Geometry check sheet. Reference: the model listing, model coordinates, mm. Round coordinates to 2 decimals unless told otherwise and drop trailing zeros. Loops run counter-clockwise (first coordinate to the right, second up) from the corner with the lowest first, then second, coordinate; pieces in that order, holes last. Notation, with made-up numbers: (-8, 78) -> (-4, 78) arc R23 cw to (-4, 99) -> close; hole circle Ø7 at (40.5, 3). An arc over 180 degrees is marked (long way). Use one line per item in the form item = value.
from build123d import *

# Parameters (mm, degrees)
EXTRUDE_2_DEPTH     = 2.5
SKETCH_2_R          = 1.5
CUT_EXTRUDE_1_DEPTH = 81.816149376


with BuildPart() as part:
    # 草图1 → 凸台-拉伸2 (new body)
    with BuildSketch(Plane(origin=(0, 0, 0), x_dir=(1, 0, 0), z_dir=(0, 1, 0))):
        Polygon((0, -30), (0, 30), (75, 30), (75, 10), (65, 10), (65, 20), (10, 20), (10, -20), (65, -20), (65, -10), (75, -10), (75, -30), align=None)
    extrude(amount=EXTRUDE_2_DEPTH)

    # 草图2 → 切除-拉伸1 (cut, through all)
    with BuildSketch(Plane(origin=(0, 0, 0), x_dir=(1, 0, 0), z_dir=(0, 1, 0))):
        with Locations(Location((5, 25, 0), (0, 0, 270))):
            Circle(SKETCH_2_R)
        with Locations(Location((70, 25, 0), (0, 0, 90))):
            Circle(SKETCH_2_R)
        with Locations(Location((70, -25, 0), (0, 0, 270))):
            Circle(SKETCH_2_R)
        with Locations(Location((5, -25, 0), (0, 0, 90))):
            Circle(SKETCH_2_R)
        with Locations(Location((37.5, -25, 0), (0, 0, 90))):
            Circle(SKETCH_2_R)
        with Locations(Location((37.5, 25, 0), (0, 0, 270))):
            Circle(SKETCH_2_R)
    extrude(amount=CUT_EXTRUDE_1_DEPTH, mode=Mode.SUBTRACT)


solid = part.part
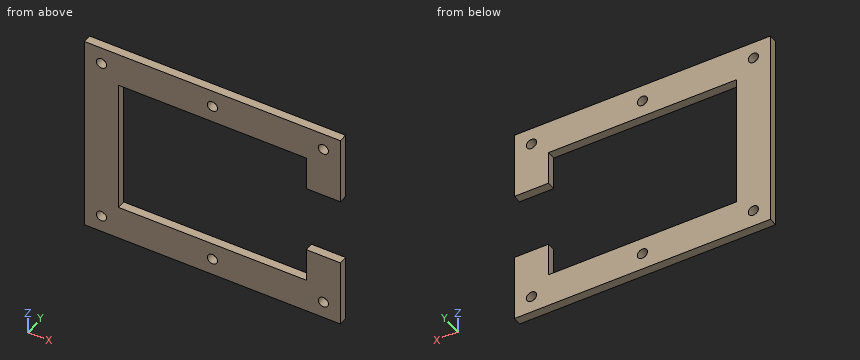
1. Section check B-B (z = -13.5). Record the boundary of the cut face in (x, y).
Return value:
outline = (0, 0) -> (10, 0) -> (10, 2.5) -> (0, 2.5) -> close; (65, 0) -> (75, 0) -> (75, 2.5) -> (65, 2.5) -> close
2. Section check D-D (z = -25). Record the boundary of the cut face in (x, y), then the cut area to 3 significant figures.
Return value:
outline = (0, 0) -> (3.5, 0) -> (3.5, 2.5) -> (0, 2.5) -> close; (6.5, 0) -> (36, 0) -> (36, 2.5) -> (6.5, 2.5) -> close; (39, 0) -> (68.5, 0) -> (68.5, 2.5) -> (39, 2.5) -> close; (71.5, 0) -> (75, 0) -> (75, 2.5) -> (71.5, 2.5) -> close
area = 165 mm2
3. Material ranges on line 1 along X through (y, z) = (1.5, -25); line 2 along Z through (x, y) = (37.5, 0.65); line 3 along X through (y, z) = (1.75, -12), recorded low to high.
Return value:
line_1 = 0 to 3.5, 6.5 to 36, 39 to 68.5, 71.5 to 75
line_2 = -30 to -26.5, -23.5 to -20, 20 to 23.5, 26.5 to 30
line_3 = 0 to 10, 65 to 75
4. Section check C-C (x = 5). Record the boundary of the cut face in (y, z).
Return value:
outline = (0, -30) -> (2.5, -30) -> (2.5, -26.5) -> (0, -26.5) -> close; (0, -23.5) -> (2.5, -23.5) -> (2.5, 23.5) -> (0, 23.5) -> close; (0, 26.5) -> (2.5, 26.5) -> (2.5, 30) -> (0, 30) -> close
5. Section check A-A (x = 66). Record the boundary of the cut face in (y, z), then the cut area to 3 significant figures.
Return value:
outline = (0, -30) -> (2.5, -30) -> (2.5, -10) -> (0, -10) -> close; (0, 10) -> (2.5, 10) -> (2.5, 30) -> (0, 30) -> close
area = 100 mm2
6. Gauge pin test, flat ends, axial feed: pin 1 (0.8 mm diameter, centred on y = 1, z = 4.5, fed in from +X); pin 2 (12 mm diameter, centred on x = 33, z = -9, fed in from -Y). Record the tip position at first contact, or that the pin passes through.
Return value:
pin_1 = 10
pin_2 = through
